Input: dimensioned drawing with shaded views. Units: mm. Origin: part minimum x, y, z. Round coordinates to 2 decimals unless told otherwise and drop trailing zeros. Order: outer loops, then holes, each group sorted by start corner. A loop starts at its lowest first (then second) coordinate and runs counter-clockwise, first axis right, second up. Notation, with made-up numbers: M 20,23.5 L 33,23.5 A29 ccw 33,57.5 Z; hole C -5,32 d4. An arc over 180 degrees is marked long. Put each result on its own line as item: value. Start each with the question number.
1) Section A-A, the plane x = 27.5. Return loops of the section in (y, z), then the cut area to 3 significant figures.
2) Material intervals for probe 1 along Y at (x, z) = (27.5, 0.85); probe 2 along Y at (x, z) = (3, 0.65); probe 3 along Y at (x, z) = (41, 1.75) (1 decimal), sorted ascending. Write a range as [from, to].
3) Section C-C, the plane x = 11. Return loops of the section in (y, z).
4) Section D-D, the plane z = 0.85. Count the separate pieces of the cut face and the enclosed holes in it, then the cut area to 3 significant figures.
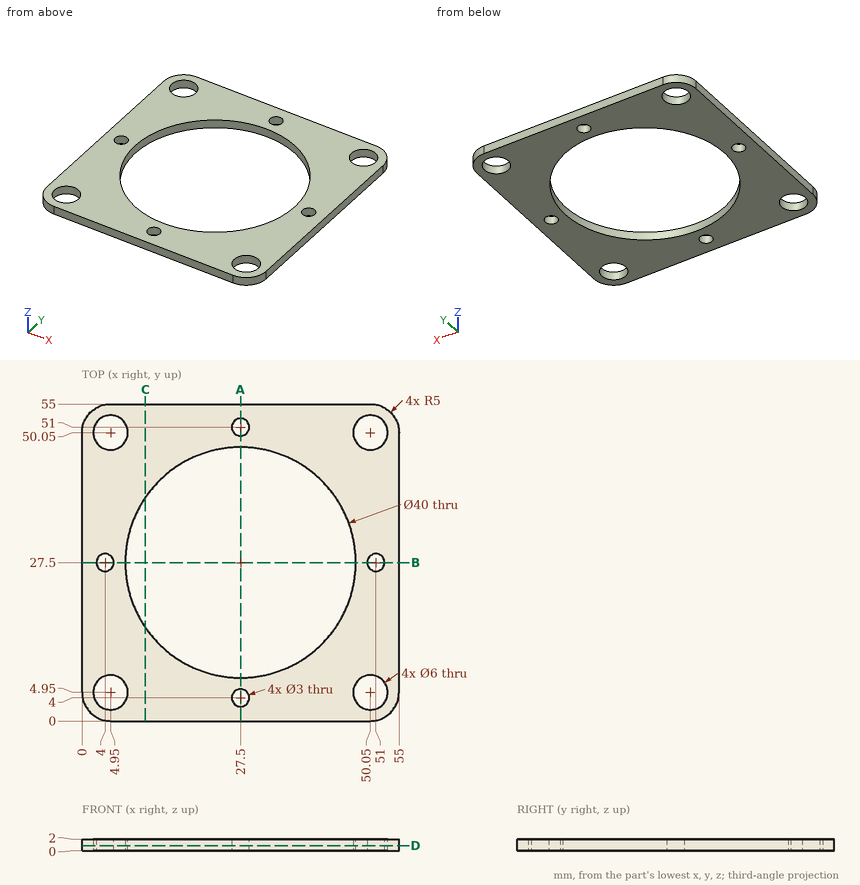
Result sheet:
1. outline: M 0,0 L 2.5,0 L 2.5,2 L 0,2 Z; M 5.5,0 L 7.5,0 L 7.5,2 L 5.5,2 Z; M 47.5,0 L 49.5,0 L 49.5,2 L 47.5,2 Z; M 52.5,0 L 55,0 L 55,2 L 52.5,2 Z
1. area: 18.0 mm2
2. probe 1: y = [0, 2.5], [5.5, 7.5], [47.5, 49.5], [52.5, 55]
2. probe 2: y = [0.42, 2.67], [7.23, 26.38], [28.62, 47.77], [52.33, 54.58]
2. probe 3: y = [0, 12.7], [42.3, 55]
3. outline: M 0,0 L 16.2,0 L 16.2,2 L 0,2 Z; M 38.8,0 L 55,0 L 55,2 L 38.8,2 Z
4. separate pieces: 1
4. enclosed holes: 9
4. area: 1,610 mm2
